The figure shows three views and two pictorial views of one solid part (mm, origin at its lowest corner). Answer the questions. A direction names the side the tool comes from. Coordinates: 2 decimals unless noted, no trailing zeros. Return JSON: item names as keys, results as strings. Group by question number.
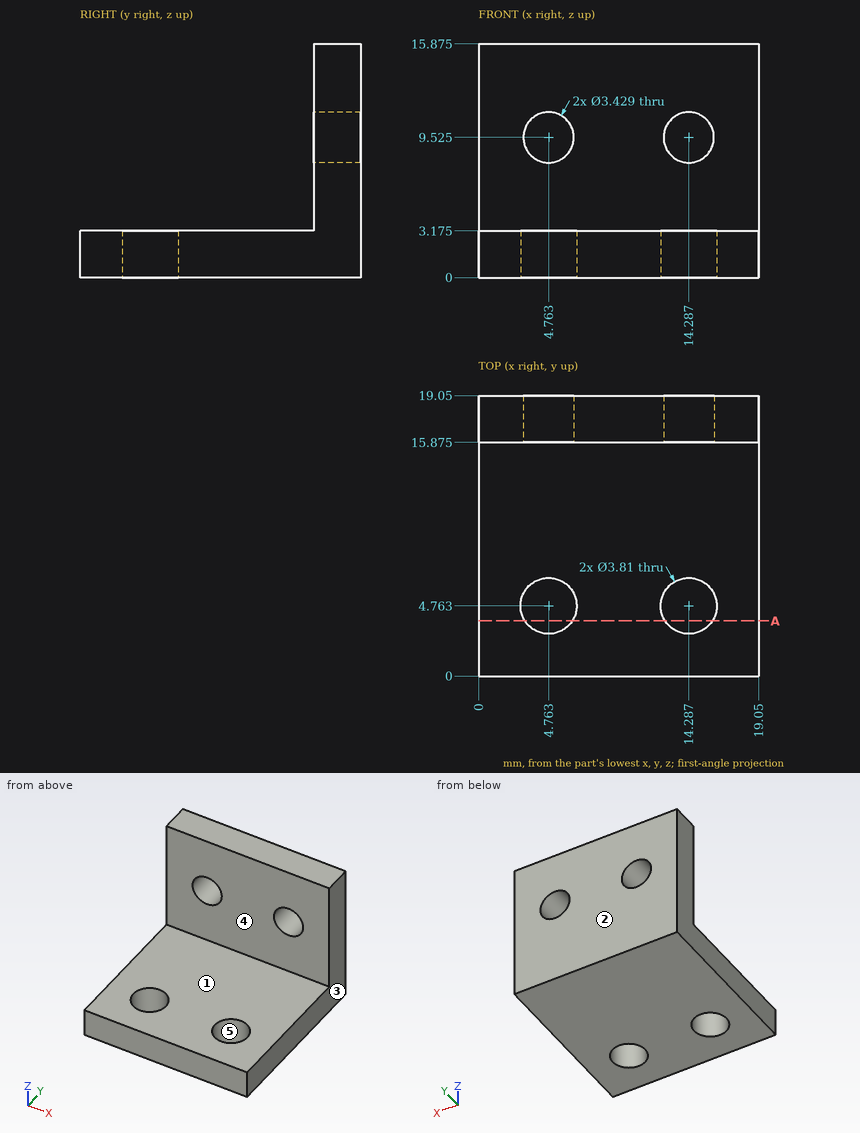
1. Find section A-A on y = 3.75. Give the number of separate pieces and of enclosed holes in the cut face.
2. Which of the six approach directions +Z, -Z, +X, -X, +Y, -Y give full straight-line access (tool end or side, diameter ignored) to the marked faces 1 and 2?
3. Straight lines are drawn through the part: L1, parallel to Z at x = 1.5, y = 11.25 (1 decimal); L2, parallel to Y at x = 5, z = 3. For each, find the intervals that lie inside material, in ascending order.
4. For a pull along X with two mould halves and no side action, classify the marked faces 3, 4 and 5 as released by +X, released by -X, zero draft, split by the parting line, or undercut.
5. Given pin 1 (2 mm diameter, centred on x = 4.76, z = 9.52, fed in from -Y); pin 2 (1 mm diameter, centred on x = 6.5, z = 4.5, fed in from -Y) (1 decimal); pin 3 (5 mm diameter, centred on x = 11, y = 8.5, fed in from +Z) (1 decimal), each flat-ended and moving along its own axis, determine where each tip first touches the part or whether it passes through.
Result:
{
 "1": {"separate pieces": "3", "enclosed holes": "0"},
 "2": {"face 1": "+Z, +X, -X, -Y", "face 2": "+Z, -Z, +X, -X, +Y"},
 "3": {"L1": "0 to 3.2", "L2": "0 to 2.87, 6.65 to 19.05"},
 "4": {"face 3": "released by +X", "face 4": "zero draft", "face 5": "undercut"},
 "5": {"pin 1": "through", "pin 2": "y = 15.9", "pin 3": "z = 3.2"}
}
